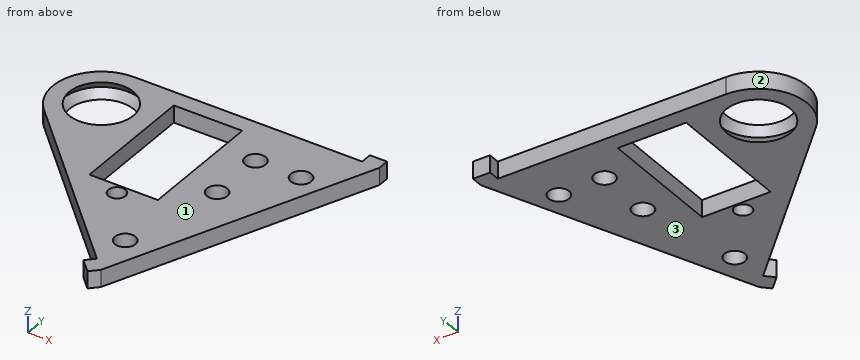
from build123d import *

# Parameters (mm, degrees)
SKETCH182_R     = 1.5
SKETCH182_W     = 22
SKETCH182_H     = 12
PAD127029_DEPTH = 17.5
SKETCH153_R     = 8
SKETCH153_R_2   = 1.8
PAD119_DEPTH    = 3


with BuildPart() as pad127029:
    # Sketch182 → Pad127029 (new body, symmetric)
    with BuildSketch(Plane(origin=(35, 160, 12), x_dir=(0, 1, 0), z_dir=(0, 0, 1))):
        with Locations((-18.25, 0)):
            Circle(SKETCH182_R)
        with Locations((-5.5, 0)):
            Rectangle(SKETCH182_W, SKETCH182_H)
    extrude(amount=PAD127029_DEPTH, both=True)


with BuildPart() as frontwheelbaseplate:
    # Sketch153 → Pad119 (new body)
    with BuildSketch(Plane(origin=(50, 160, 8.5), x_dir=(1, 0, 0), z_dir=(0, 0, 1))):
        with BuildLine():
            ThreePointArc((6.010433, -6.010382), (7.852969, 3.252826), (0, 8.5))
            Line((0, 8.5), (-40, 8.5))
            Line((-40, 8.5), (-40, 10.5))
            Line((-40, 10.5), (-43, 10.5))
            Line((-43, 10.5), (-43, 8.5))
            Line((-43, 8.5), (-24.395158, -36.415973))
            Line((-24.395158, -36.415973), (-22.980945, -37.830187))
            Line((-22.980945, -37.830187), (-20.859624, -35.708867))
            Line((-20.859624, -35.708867), (-22.273838, -34.294653))
            Line((6.010433, -6.010382), (-22.273838, -34.294653))
        make_face()
        Circle(SKETCH153_R, mode=Mode.SUBTRACT)
        with Locations((-27, 0)):
            Circle(SKETCH153_R_2, mode=Mode.SUBTRACT)
        with Locations((-27, -10)):
            Circle(SKETCH153_R_2, mode=Mode.SUBTRACT)
        with Locations((-23, -28)):
            Circle(SKETCH153_R_2, mode=Mode.SUBTRACT)
        with Locations((-35, 0)):
            Circle(SKETCH153_R_2, mode=Mode.SUBTRACT)
    extrude(amount=PAD119_DEPTH)


with BuildPart() as steeringbaseplate:
    # Sketch151 → Revolution007 (revolve)
    with BuildSketch(Plane(origin=(50, 160, 10), x_dir=(1, 0, 0), z_dir=(0, -1, 0))):
        Polygon((5.634953, 1.5), (6.685264, 0), (5.634953, -1.5), (8, -1.5), (8, 1.5), align=None)
    revolve(axis=Axis((50, 160, 10), (0, 0, 1)))

    # Fusion004020020: union FrontWheelBasePlate
    add(frontwheelbaseplate.part)

    # Cut007019020: cut Pad127029
    add(pad127029.part, mode=Mode.SUBTRACT)


with BuildPart() as part_mirroring011:
    # Part__Mirroring011: instance of SteeringBasePlate
    add(steeringbaseplate.part.mirror(Plane(origin=(0, 0, 0), x_dir=(0, -1, 0), z_dir=(1, 0, 0))))


solid = part_mirroring011.part
Input: part model. Units: mm. Frame: model coordinates. Face numbers are marked on the shaded views. Coordinates: 2 decimals unless noted, no trailing zeros. Loops run counter-clockwise (first coordinate to the right, second up) from the corner with the lowest first, then second, coordinate; pieces in that order, holes last.
Q1. Cut plane A-A (y = 150). Output: boundary loops of the cut face in (x, z).
Q2. Cut plane B-B (z = 10.7). Output: boundary loops of the cut face in (x, y).
Q3. Contact query for flat-ended pins moving along their axis: pin 1 (1 mm diameter, centred on y = 169.5, z = 10.5, fed in from -X); pin 2 (1.5 mm diameter, centred on x = -31.5, y = 155.5, fed in from -Z); pin 3 (0.9 mm diameter, centred on x = -36, z = 9.5, fed in from +Y); pin 4 (6 mm diameter, centred on x = -23, y = 160, fed in from -Z). Output: stop coordinate, or through.
Q4. Cut plane C-C (x = -37.5). Output: boundary loops of the cut face in (y, z).
Q5. Material intervals for line 1 (X direction, y = 163, z = 9.95); line 2 (X direction, y = 156, z = 9.1); line 3 (Y direction, x = -34, z = 9.25), sorted ascending.
Q6. Draft query along Z for the marked faces 1, 2 and 3. Return one class per face: +Z half, -Z half, draft (parallel to the pull), parting line (faces both ways), or undercut.
Q7. Cut plane D-D (y = 141.75). Output: boundary loops of the cut face in (x, z), then the cut area to 3 significant figures.
Working result:
1. outline: (-52.02, 8.5) - (-41, 8.5) - (-41, 11.5) - (-52.02, 11.5) - close; (-29, 8.5) - (-24.8, 8.5) - (-24.8, 11.5) - (-29, 11.5) - close; (-21.2, 8.5) - (-14.66, 8.5) - (-14.66, 11.5) - (-21.2, 11.5) - close
2. outline: (-56.01, 153.99) - (-27.73, 125.71) - (-29.14, 124.29) - (-27.02, 122.17) - (-25.6, 123.58) - (-7, 168.5) - (-7, 170.5) - (-10, 170.5) - (-10, 168.5) - (-50, 168.5) arc R8.5 ccw to start; hole circle Ø12.39 at (-50, 160); hole (-41, 143.5) - (-29, 143.5) - (-29, 165.5) - (-41, 165.5) - close; hole circle Ø3 at (-35, 141.75); hole circle Ø3.6 at (-27, 132); hole circle Ø3.6 at (-23, 150); hole circle Ø3.6 at (-23, 160); hole circle Ø3.6 at (-15, 160)
3. pin 1: stops at x = -10
3. pin 2: passes through
3. pin 3: stops at y = 168.5
3. pin 4: stops at z = 8.5
4. outline: (135.48, 8.5) - (143.5, 8.5) - (143.5, 11.5) - (135.48, 11.5) - close; (165.5, 8.5) - (168.5, 8.5) - (168.5, 11.5) - (165.5, 11.5) - close
5. line 1: x = -57.95 to -55.94, -44.06 to -41, -29 to -9.28
5. line 2: x = -57.5 to -54.55, -45.45 to -41, -29 to -12.18
5. line 3: y = 131.98 to 140.63, 142.87 to 143.5, 165.5 to 168.5
6. face 1: +Z half
6. face 2: draft
6. face 3: -Z half
7. outline: (-43.77, 8.5) - (-36.5, 8.5) - (-36.5, 11.5) - (-43.77, 11.5) - close; (-33.5, 8.5) - (-18.08, 8.5) - (-18.08, 11.5) - (-33.5, 11.5) - close
7. area: 68.1 mm2
